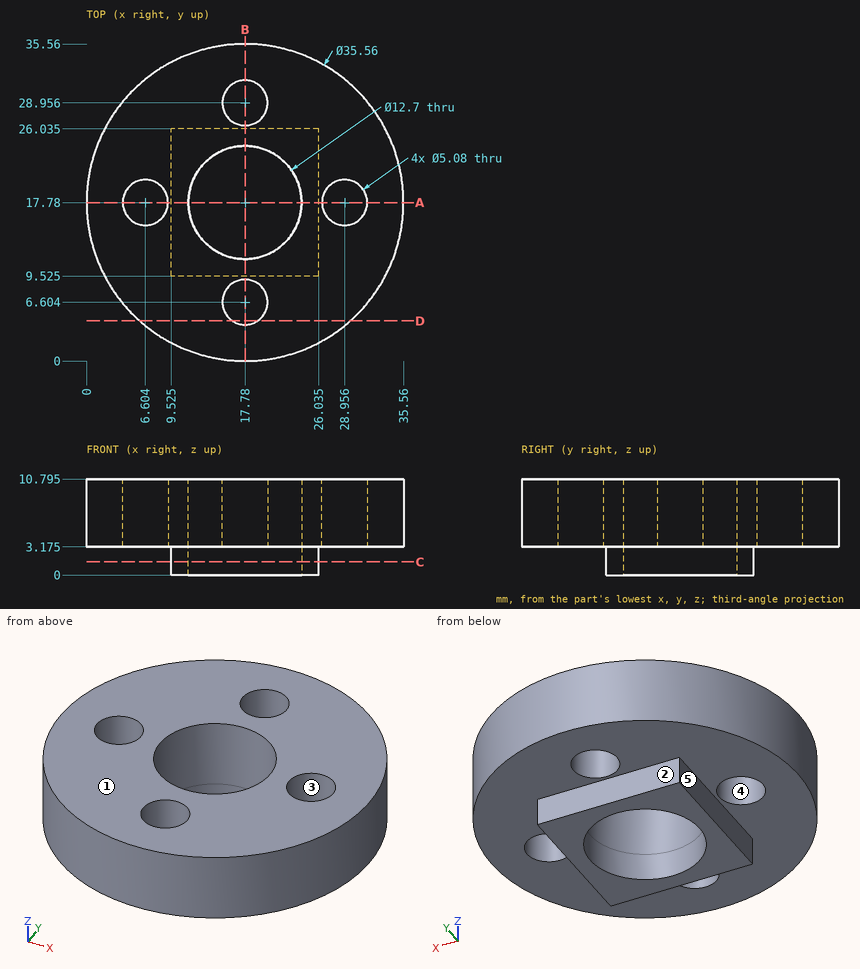
Here's the drawing with two shaded views (mm, measured from the low corner). I have some questions. A direction names the side the tool comes from. Coordinates: 2 decimals unless noted, no trailing zeros. Order: outer loops, then holes, each group sorted by start corner. A loop starts at its lowest first (then second) coordinate and runs counter-clockwise, first axis right, second up. Notation, with made-up numbers: M 35.25,0.5 L 80.25,0.5 A27 ccw 80.25,28.5 Z; hole C -35.5,-24 d6. An arc over 180 degrees is marked long. Answer as CSV lines item,"result".
Item 1: For pin 1 (3.5 mm diameter, centred on x = 15, z = 1.5, fed in from +Y); pin 2 (4 mm diameter, centred on y = 6, z = 5, fed in from -X); pin 3 (3.5 mm diameter, centred on y = 14.5, z = 2, fed in from +X), each with a flat end and sliding along its axis, tell me the tip position at first contact or that it passes through.
Results found:
pin 1,"y = 35.41"
pin 2,"x = 2.93"
pin 3,"x = 35.45"
Item 2: We'd pull the mould along Y, two halves only. Please class the marked faces 1, 2 and 3: +Y half, -Y half, draft (parallel to the pull), parting line (faces both ways), or undercut.
Results found:
face 1,"draft"
face 2,"+Y half"
face 3,"undercut"
Item 3: Imagine slicing it at D-D on y = 4.5. Write out the boundary of the cut face in (x, z) (3 decimals), plus the area to 3 significant figures.
Results found:
outline,"M 5.958,3.175 L 16.357,3.175 L 16.357,10.795 L 5.958,10.795 Z; M 19.203,3.175 L 29.602,3.175 L 29.602,10.795 L 19.203,10.795 Z"
area,"158 mm2"
Item 4: Imagine slicing it at A-A on y = 17.78. Write out the boundary of the cut face in (x, z) (3 decimals).
Results found:
outline,"M 0,3.175 L 4.064,3.175 L 4.064,10.795 L 0,10.795 Z; M 9.144,3.175 L 9.525,3.175 L 9.525,0 L 11.43,0 L 11.43,10.795 L 9.144,10.795 Z; M 24.13,0 L 26.035,0 L 26.035,3.175 L 26.416,3.175 L 26.416,10.795 L 24.13,10.795 Z; M 31.496,3.175 L 35.56,3.175 L 35.56,10.795 L 31.496,10.795 Z"
Item 5: Imagine slicing it at C-C on z = 1.5. Write out the boundary of the cut face in (x, y) (3 decimals), plus the area to 3 significant figures.
Results found:
outline,"M 9.525,9.525 L 26.035,9.525 L 26.035,26.035 L 9.525,26.035 Z; hole C 17.78,17.78 d12.7"
area,"146 mm2"
Item 6: If I drill on line 1 (Y direction, x = 17.78, z = 5); line 2 (Y direction, x = 19.5, z = 8); line 3 (Y direction, x = 17.78, z = 1.35) (3 decimals), over which ranges is the centre line in solid material (lowest first)?
Results found:
line 1,"0 to 4.06, 9.14 to 11.43, 24.13 to 26.42, 31.5 to 35.56"
line 2,"0.08 to 4.73, 8.47 to 11.67, 23.89 to 27.09, 30.83 to 35.48"
line 3,"9.525 to 11.43, 24.13 to 26.035"
Item 7: On a 3-axis mill with a long thin cutter (end or side, diameter ignored), from which of +Z, -Z, +X, -X, +Y, -Y can I reach the whole of each face in a straight line? I mean the marked faces 4 and 5. Say none if no direction works.
Results found:
face 4,"+Z, -Z"
face 5,"-Z, -X, +Y, -Y"
